Geometry: final body of the model. Coordinates: model frame, mm. Face numbers are marked on the shaded views. Give positions to 0.01 mm unless a question says otherwise; leave off trailing zeros. Loops run counter-clockwise (first coordinate to the right, second up) from the corner with the lowest first, then second, coordinate; pieces in that order, holes last. Notation, with made-up numbers: (61.5, 68) - (101.5, 68) arc R34 ccw to (101.5, 101) - close; hole circle Ø9 at (26, 65). An arc over 180 degrees is marked (long way). Answer in a Markdown table with one row per item.
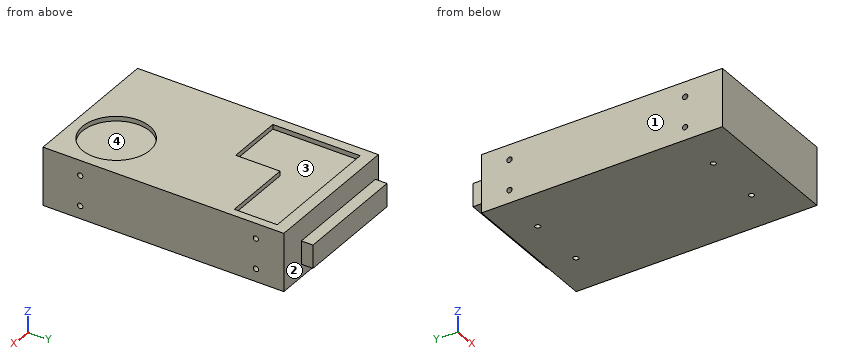
from build123d import *

# Parameters (mm, degrees)
SKETCH1_W           = 124
SKETCH1_H           = 225
BOSS_EXTRUDE1_DEPTH = 50
SKETCH2_W           = 142.142792237
SKETCH2_H           = 18
CUT_EXTRUDE1_DEPTH  = 50
SKETCH3_W           = 97
SKETCH3_H           = 20
BOSS_EXTRUDE2_DEPTH = 10
SKETCH4_R           = 29
CUT_EXTRUDE3_DEPTH  = 4
SKETCH5_R           = 2.25
CUT_EXTRUDE4_DEPTH  = 15
SKETCH6_R           = 2.25
CUT_EXTRUDE5_DEPTH  = 175.734799053


with BuildPart() as part:
    # Sketch1 → Boss-Extrude1 (new body)
    with BuildSketch(Plane.XY):
        Rectangle(SKETCH1_W, SKETCH1_H)
    extrude(amount=BOSS_EXTRUDE1_DEPTH)

    # Sketch2 → Cut-Extrude1 (cut)
    with BuildSketch(Plane.XY.offset(50)):
        with Locations((-0.947920956, 103.5)):
            Rectangle(SKETCH2_W, SKETCH2_H)
    extrude(amount=-CUT_EXTRUDE1_DEPTH, mode=Mode.SUBTRACT)

    # Sketch3 → Boss-Extrude2 (add)
    with BuildSketch(Plane(origin=(0, 94.5, 0), x_dir=(1, 0, 0), z_dir=(0, 1, 0))):
        with Locations((-9.5, -21)):
            Rectangle(SKETCH3_W, SKETCH3_H)
    extrude(amount=BOSS_EXTRUDE2_DEPTH)

    # Sketch4 → Cut-Extrude3 (cut)
    with BuildSketch(Plane.XY.offset(50)):
        with Locations((23.52502673, -74.82534643)):
            Circle(SKETCH4_R)
        Polygon((-53.556975746, 84.343983357), (55.058573197, 84.343983357), (55.058573197, 47.30457957), (-5.005324836, 47.30457957), (-5.005324836, 9.264110816), (-53.556975746, 9.264110816), align=None)
    extrude(amount=-CUT_EXTRUDE3_DEPTH, mode=Mode.SUBTRACT)

    # Sketch5 → Cut-Extrude4 (cut)
    with BuildSketch(Plane(origin=(0, 0, 0), x_dir=(-1, 0, 0), z_dir=(0, 0, -1))):
        with Locations((-25, 70.5)):
            Circle(SKETCH5_R)
        with Locations((25, 70.5)):
            Circle(SKETCH5_R)
        with Locations((25, -80.5)):
            Circle(SKETCH5_R)
        with Locations((-25, -80.5)):
            Circle(SKETCH5_R)
    extrude(amount=-CUT_EXTRUDE4_DEPTH, mode=Mode.SUBTRACT)

    # Sketch6 → Cut-Extrude5 (cut, through all)
    with BuildSketch(Plane.ZY.offset(62)):
        with Locations(Location((11, 70.5, 0), (0, 0, 270))):
            Circle(SKETCH6_R)
        with Locations(Location((37, 70.5, 0), (0, 0, 270))):
            Circle(SKETCH6_R)
        with Locations(Location((37, -80.5, 0), (0, 0, 270))):
            Circle(SKETCH6_R)
        with Locations(Location((11, -80.5, 0), (0, 0, 270))):
            Circle(SKETCH6_R)
    extrude(amount=-CUT_EXTRUDE5_DEPTH, mode=Mode.SUBTRACT)


solid = part.part
Q1. Cut plane A-A (y = 70.5). Give the number of separate pieces and of enclosed holes in the cut face, and give its area (3 significant figures).
Check values:
| item | result |
|---|---|
| separate pieces | 5 |
| enclosed holes | 0 |
| area | 4,560 mm² |
Q2. Draft query along X for the marked faces 1, 2, 3 and 4. Return one class per face: pulls with the +X half, pulls with the -X half, needs draft (parallel to the pull), parting line crosses it, or undercut.
Check values:
| item | result |
|---|---|
| face 1 | pulls with the -X half |
| face 2 | needs draft |
| face 3 | undercut |
| face 4 | undercut |
Q3. First-contact query: pin 1 (4 mm diameter, centred on x = -25, y = 70.5, fed in from +Z); pin 2 (5 mm diameter, centred on x = 44, z = 41.5, fed in from +Y); pin 3 (3 mm diameter, centred on y = 101, z = 16, fed in from -X); pin 4 (3.5 mm diameter, centred on y = 70.5, z = 11, fed in from -X). Flat tips, straight axial feed; report the tip coordinate or a pass-through.
Check values:
| item | result |
|---|---|
| pin 1 | z = 46 |
| pin 2 | y = 94.5 |
| pin 3 | x = -58 |
| pin 4 | through |
Q4. Cut plane C-C (y = 39.5). Output: boundary loops of the cut face in (x, z), and give its area (3 significant figures).
Check values:
| item | result |
|---|---|
| outline | (-62, 0) - (62, 0) - (62, 50) - (-5.01, 50) - (-5.01, 46) - (-53.56, 46) - (-53.56, 50) - (-62, 50) - close |
| area | 6,010 mm² |
Q5. Cut plane B-B (x = -10.5). Output: boundary loops of the cut face in (y, z), and give its area (3 significant figures).
Check values:
| item | result |
|---|---|
| outline | (-112.5, 0) - (94.5, 0) - (94.5, 11) - (104.5, 11) - (104.5, 31) - (94.5, 31) - (94.5, 50) - (84.34, 50) - (84.34, 46) - (9.26, 46) - (9.26, 50) - (-112.5, 50) - close; hole circle Ø4.5 at (-80.5, 11); hole circle Ø4.5 at (-80.5, 37); hole circle Ø4.5 at (70.5, 11); hole circle Ø4.5 at (70.5, 37) |
| area | 10,200 mm² |
Q6. Material intervals for line 1 along Y through (x, z) = (-25, 14); line 2 along Z through (x, y) = (34.5, -80.5); line 3 along Y through (x, z) = (25, 3), sorted ascending.
Check values:
| item | result |
|---|---|
| line 1 | -112.5 to -82.75, -78.25 to 68.25, 72.75 to 104.5 |
| line 2 | 0 to 8.75, 13.25 to 34.75, 39.25 to 46 |
| line 3 | -112.5 to -82.75, -78.25 to 68.25, 72.75 to 94.5 |
